```python
from build123d import *

# Parameters (mm, degrees)
F0_R     = 1.5
F1_DEPTH = 1
F2_W     = 20
F2_H     = 23
F3_DEPTH = 4


with BuildPart() as f1:
    # F0 (on Top) → F1 (new body)
    with BuildSketch(Plane.XY):
        with BuildLine():
            Line((16, 18), (-16, 18))
            ThreePointArc((-16, 18), (-17.414214, 17.414214), (-18, 16))
            Line((-18, 16), (-18, -16))
            ThreePointArc((-18, -16), (-17.414214, -17.414214), (-16, -18))
            Line((-16, -18), (16, -18))
            ThreePointArc((16, -18), (17.414214, -17.414214), (18, -16))
            Line((18, -16), (18, 16))
            ThreePointArc((18, 16), (17.414214, 17.414214), (16, 18))
        make_face()
        with Locations((-15.5, -15.5)):
            Circle(F0_R, mode=Mode.SUBTRACT)
        with Locations((15.5, -15.5)):
            Circle(F0_R, mode=Mode.SUBTRACT)
        with Locations((-15.5, 15.5)):
            Circle(F0_R, mode=Mode.SUBTRACT)
        with Locations((15.5, 15.5)):
            Circle(F0_R, mode=Mode.SUBTRACT)
    extrude(amount=F1_DEPTH)

    # F2 (on face) → F3 (join)
    with BuildSketch(Plane.XY.offset(1)):
        Rectangle(F2_W, F2_H)
    extrude(amount=F3_DEPTH)


solid = f1.part
```
Verification items for the finished model (mm, model axes). A direction names the side the tool comes from. Give positions to 0.01 mm unless a question says otherwise; leave off trailing zeros. Order: outer loops, then holes, each group sorted by start corner. A loop starts at its lowest first (then second) coordinate and runs counter-clockwise, first axis right, second up. Notation, with made-up numbers: M 14.5,-29.75 L 56.5,-29.75 A18 ccw 56.5,-9.75 Z; hole C 21,65 d2. An arc over 180 degrees is marked long. Answer in a Markdown table with one row per item. Add a question column.
Item 1: Gauge pin test, flat ends, axial feed: pin 1 (2.5 mm diameter, centred on x = -15.5, y = 15.5, fed in from -Z); pin 2 (2 mm diameter, centred on y = -0.5, z = 3.5, fed in from +X); pin 3 (3 mm diameter, centred on y = -2.5, z = 3, fed in from -X). Record the tip position at first contact, or that the pin passes through.
Item 2: Section check A-A, the plane y = 15.5. Enter the section's corners in (x, z), and give its area (3 significant figures).
Item 3: Scan lines: probe 1 along Y at (x, z) = (15.5, 0.2); probe 2 along X at (y, z) = (-2, 1.9); probe 3 along Z at (x, y) = (12, 5). Record each from-to range of solid material in increasing order. Write a range as from..to.
Item 4: Section check D-D, the plane y = 7.5. Enter the section's corners in (x, z).
Item 5: Mould release check, pull along X, two halves, no side actions. Record for faces 4 (the flat face through (18, -0.2, 0.5)), 5 (the cylindrical face through (-17, 15.57, 0.49)), 6 (the flat face through (0, 0, 0)): released by +X, released by -X, zero draft, split by the parting line, or undercut.
Item 6: Tool access check on faces 1 (the flat face through (0, 11.5, 3)), 2 (the flat face through (10, 0, 3)), 3 (the flat face through (-10, 0, 3)). Record the directions out of +Z, -Z, +X, -X, +Y, -Y that give a thin tool (end or side, any length) a straight path to the whole face; none if there is none.
Item 7: Section check C-C, the plane z = 0.45. Enter the section's corners in (x, y).
Filled sheet:
| question | item | result |
|---|---|---|
| 1 | pin 1 | passes through |
| 1 | pin 2 | stops at x = 10 |
| 1 | pin 3 | stops at x = -10 |
| 2 | outline | M -18,0 L -17,0 L -17,1 L -18,1 Z; M -14,0 L 14,0 L 14,1 L -14,1 Z; M 17,0 L 18,0 L 18,1 L 17,1 Z |
| 2 | area | 30.0 mm^2 |
| 3 | probe 1 | y = -18..-17, -14..14, 17..18 |
| 3 | probe 2 | x = -10..10 |
| 3 | probe 3 | z = 0..1 |
| 4 | outline | M -18,0 L 18,0 L 18,1 L 10,1 L 10,5 L -10,5 L -10,1 L -18,1 Z |
| 5 | face 4 | released by +X |
| 5 | face 5 | undercut |
| 5 | face 6 | zero draft |
| 6 | face 1 | +Z, +X, -X, +Y |
| 6 | face 2 | +Z, +X, +Y, -Y |
| 6 | face 3 | +Z, -X, +Y, -Y |
| 7 | outline | M -18,-16 A2 ccw -16,-18 L 16,-18 A2 ccw 18,-16 L 18,16 A2 ccw 16,18 L -16,18 A2 ccw -18,16 Z; hole C -15.5,-15.5 d3; hole C -15.5,15.5 d3; hole C 15.5,-15.5 d3; hole C 15.5,15.5 d3 |
